Autodesk Inventor part; units mm, degrees
ref_plane "YZ Plane" through (0, 0, 0) normal (1, 0, 0) x (0, 1, 0)
ref_plane "XZ Plane" through (0, 0, 0) normal (0, 1, 0) x (-1, 0, 0)
ref_plane "XY Plane" through (0, 0, 0) normal (0, 0, 1) x (1, 0, 0)
sketch "Sketch1" plane through (0, 0, 0) normal (0, 0, 1) x (1, 0, 0)
  circle A0 centre (-1.6749, 21.9538) radius 2.1844
  circle A1 centre (-1.6749, -3.4462) radius 2.1844
  line L0 (23.7251, 85.917) -> (23.7251, -92.3462)
  line L1 (-28.6624, -92.3462) -> (-28.6624, 91.8038)
  line L2 (17.3751, 64.8163) -> (20.5501, 63.2288)
  line L3 (20.5501, 63.2288) -> (20.5501, 10.8413)
  line L4 (20.5501, 10.8413) -> (17.3751, 12.4288)
  line L5 (17.3751, 12.4288) -> (17.3751, 64.8163)
  line L6 (20.5501, 75.9288) -> (17.3751, 83.8663)
  line L7 (20.5501, 90.2163) -> (20.5501, 75.9288)
  line L8 (17.6728, 70.1741) -> (14.4978, 78.1116)
  line L9 (17.3751, 83.8663) -> (20.5501, 90.2163)
  line L10 (-18.3436, 12.4288) -> (-15.1686, 4.4913)
  line L11 (-15.9624, 17.1913) -> (-12.7874, 9.2538)
  line L12 (-15.9624, 17.1913) -> (14.4978, 78.1116)
  line L13 (-23.1061, 2.9038) -> (-19.9311, -5.0337)
  line L14 (-23.1061, 2.9038) -> (-23.1061, -11.3837)
  line L15 (-20.7249, 7.6663) -> (-18.3436, 12.4288)
  line L16 (-15.1686, 4.4913) -> (-17.5499, -0.2712)
  line L17 (-19.9311, -5.0337) -> (-23.1061, -11.3837)
  line L18 (11.8546, 90.2163) -> (11.8546, 82.3502)
  line L19 (11.8546, 90.2163) -> (-6.4374, 90.2163)
  line L20 (11.8546, 82.3502) -> (-6.4374, 45.7663)
  line L21 (0.5095, 17.1913) -> (-6.4374, 4.4913)
  line L22 (12.6126, -19.3212) -> (0.5095, 17.1913)
  line L23 (-10.761, -3.4129) -> (-19.992, -30.0754)
  line L24 (-19.992, -30.0754) -> (-17.153, -52.6587)
  line L25 (-17.153, -52.6587) -> (-9.533, -62.1837)
  line L26 (-7.1105, -44.6247) -> (-9.533, -30.0754)
  line L27 (-9.533, -30.0754) -> (-1.9594, -8.2002)
  line L28 (-5.9563, -5.5321) -> (-10.761, -3.4129)
  line L29 (20.5501, -79.2004) -> (20.5501, -92.3462)
  line L30 (6.9368, -62.1837) -> (4.2652, -64.3209)
  line L31 (-1.5433, -71.7065) -> (14.9685, -92.3462)
  arc A2 (-1.5433, -71.7065) -> (3.0742, -66.8586) centre (-1.6875, -66.9462) ccw
  circle A3 centre (-1.6875, -66.9462) radius 2.1844
  arc A4 (4.2652, -64.3209) -> (3.0742, -66.8586) centre (6.2486, -66.8002) ccw
  line L32 (20.5501, -79.2004) -> (6.9368, -62.1837)
  line L33 (23.7251, -92.3462) -> (20.5501, -92.3462)
  circle A5 centre (-1.6749, -54.2462) radius 2.1844
  arc A6 (-4.5442, -50.4451) -> (-5.5294, -57.0433) centre (-1.6749, -54.2462) ccw
  line L34 (-9.533, -62.1837) -> (-5.8225, -59.2153)
  line L35 (0.5075, -54.1513) -> (0.5095, -54.1497)
  line L36 (0.5095, -54.1497) -> (0.5073, -54.1469)
  line L37 (-4.2611, -48.1864) -> (-7.1105, -44.6247)
  arc A7 (-4.5442, -50.4451) -> (-4.2611, -48.1864) centre (-5.5007, -49.1781) ccw
  arc A8 (-5.8225, -59.2153) -> (-5.5294, -57.0433) centre (-6.8142, -57.9757) ccw
  arc A9 (-4.5324, 25.7638) -> (-6.4374, 21.9538) centre (-1.6749, 21.9538) ccw
  line L38 (17.6728, 70.1741) -> (-4.5324, 25.7638)
  line L39 (-6.4374, 21.9538) -> (-12.7874, 9.2538)
  line L40 (-6.4374, 4.4913) -> (-3.5794, 0.9189)
  line L41 (2.1657, -6.2625) -> (12.6126, -19.3212)
  arc A10 (2.1657, -6.2625) -> (-3.5794, 0.9189) centre (-1.6749, -3.4462) ccw
  arc A11 (-5.9563, -5.5321) -> (-1.9594, -8.2002) centre (-1.6749, -3.4462) ccw
  line L42 (14.9685, -92.3462) -> (44.3118, -92.3462) construction
  line L43 (-2.7748, -92.3462) -> (14.9685, -92.3462)
  line L44 (-28.6624, -92.3462) -> (-23.2121, -92.3462)
  line L45 (-18.5725, -92.3462) -> (-28.6624, -92.3462)
  line L46 (-20.7249, 7.6663) -> (-17.5499, -0.2712)
  line L47 (-28.6624, 98.1538) -> (-28.6624, 101.3288)
  line L48 (-19.1374, 101.3288) -> (11.0251, 101.3288)
  line L49 (23.7251, 90.2163) -> (23.7251, 85.917)
  line L50 (11.0251, 101.3288) -> (23.7251, 90.2163)
  arc A12 (-19.1374, 101.3288) -> (-28.6624, 91.8038) centre (-19.1374, 91.8038) ccw
  arc A13 (-6.4374, 74.6137) -> (-6.4374, 83.5939) centre (-8.0249, 79.1038) ccw
  circle A14 centre (-8.0249, 79.1038) radius 2.1844
  line L51 (-6.4374, 90.2163) -> (-6.4374, 83.5939)
  line L52 (-6.4374, 74.6137) -> (-6.4374, 45.7663)
  line L53 (-18.5725, -92.3462) -> (-15.3911, -92.3462)
  line L54 (-15.3911, -92.3462) -> (-15.3911, -76.5759)
  line L55 (-15.3911, -76.5759) -> (-2.7748, -92.3462)
  point P0 (0, 0)
  point P1 (2.838, -65.4627)
  point P2 (-4.4495, -58.1169)
  point P3 (-3.0588, -49.6892)
  dimension "d0" = 4.3688
  dimension "d1" = 4.3688
  dimension "d3" = 9.525
  dimension "d4" = 4.3688
  dimension "d5" = 3.175
  dimension "d6" = 9.525
  dimension "d7" = 1.5875
  dimension "d8" = 9.525
  dimension "d14" = 3.175
  dimension "d15" = 9.525
  dimension "d18" = 9.525
  dimension "d19" = 4.3688
  dimension "d20" = 3.1814
extrude "Extrusion1" add sketch "Sketch1" along normal blind 1.5875
equation "\"BendRadius\" = Thickness"
equation "\"BendReliefWidth\" = Thickness"
equation "\"BendReliefDepth\" = 0.5 * Thickness"
equation "\"CornerReliefSize\" = 4 * Thickness"
equation "\"MinimumRemnant\" = 2 * Thickness"
equation "\"TransitionRadius\" = BendRadius"
equation "\"JacobiRadiusSize\" = BendRadius"
equation "\"GapSize\" = Thickness"
properties part number "sideplate" material "Acetal Resin, White"
Geometry check sheet. Reference: the model listing, model coordinates, mm. A direction names the side the tool comes from. Round coordinates to 2 decimals unless told otherwise and drop trailing zeros. Loops run counter-clockwise (first coordinate to the right, second up) from the corner with the lowest first, then second, coordinate; pieces in that order, holes last. Notation, with made-up numbers: (38, -17.75) - (96, -17.75) arc R19 ccw to (96, 5.25) - close; hole circle Ø11 at (-7, 30). An arc over 180 degrees is marked (long way). Write each question's results on one line, items separated by ' | '. Start each with the question number.
Q1. Access from +Z, -Z, +X, -X, +Y, -Y to the whole of each face (thin tool, end or side, straight path). Record for faces 1 (the flat face through (-5.8, -19.29, 0.78)), 2 (the flat face through (-9, 6, 1.588)).
Q2. Thickness scan on line 1 (X direction, y = -13.5, z = 1); line 2 (X direction, y = 84, z = 0.35); line 3 (Y direction, x = 13, z = 0.9). Record the ranges inside material, lowest first. Write a range as [from, to].
Q3. Cross-section at D-D on z = 0.7. State how many separate pieces and enclosed holes the cut face has, and give its area (3 significant figures).
Q4. Cross-section at A-A on y = 15. Enter the section's corners in (x, z), and give its area (3 significant figures).
Q5. Release check for a two-part mould opening along X. For faces 3 (the flat face through (17.286, 95.85, 0.783)), 4 (the flat face through (-13.4, -57.35, 0.78)), 5 (the cylindrical face through (-25.95, 98.46, 0.78)) record: +X half, -X half, draft (parallel to the pull), parting line (faces both ways), or undercut.
Q6. Cross-section at B-B on y = 72.5. Enter the section's corners in (x, z), and give its area (3 significant figures).
Q7. Cross-section at C-C on y = -37. Enter the section's corners in (x, z), and give its area (3 significant figures).
Answers below:
1) face 1: +Z, -Z | face 2: +Z, +X, -X, +Y, -Y
2) line 1: x = [-28.66, -14.25], [-3.79, 7.96], [10.68, 23.73] | line 2: x = [-28.66, -6.44], [11.85, 17.44], [20.55, 23.73] | line 3: y = [-92.35, -89.89], [-69.76, 60.83], [75.12, 99.6]
3) separate pieces: 1 | enclosed holes: 13 | area: 7,650 mm²
4) outline: (-28.66, 0) - (-15.09, 0) - (-15.09, 1.59) - (-28.66, 1.59) - close; (-9.91, 0) - (-0.69, 0) - (-0.69, 1.59) - (-9.91, 1.59) - close; (1.24, 0) - (17.38, 0) - (17.38, 1.59) - (1.24, 1.59) - close; (20.55, 0) - (23.73, 0) - (23.73, 1.59) - (20.55, 1.59) - close | area: 66.9 mm²
5) face 3: +X half | face 4: undercut | face 5: -X half
6) outline: (-28.66, 0) - (-6.44, 0) - (-6.44, 1.59) - (-28.66, 1.59) - close; (6.93, 0) - (11.69, 0) - (11.69, 1.59) - (6.93, 1.59) - close; (16.74, 0) - (23.73, 0) - (23.73, 1.59) - (16.74, 1.59) - close | area: 53.9 mm²
7) outline: (-28.66, 0) - (-19.12, 0) - (-19.12, 1.59) - (-28.66, 1.59) - close; (-8.38, 0) - (23.73, 0) - (23.73, 1.59) - (-8.38, 1.59) - close | area: 66.1 mm²
